from build123d import *

# Parameters (mm, degrees)
F0_R     = 2
F1_DEPTH = 4
F2_W     = 12
F2_H     = 4
F3_DEPTH = 4
F4_W     = 12
F4_H     = 20
F4_R     = 2
F5_DEPTH = 4


with BuildPart() as f1:
    # F0 (on Front) → F1 (new body)
    with BuildSketch(Plane.XZ):
        Polygon((-28, -4), (28, -4), (28, 4), (28, 16), (16, 16), (16, 4), (-16, 4), (-16, 16), (-28, 16), (-28, 4), align=None)
        with Locations((-24, 0)):
            Circle(F0_R, mode=Mode.SUBTRACT)
        Circle(F0_R, mode=Mode.SUBTRACT)
        with Locations((24, 0)):
            Circle(F0_R, mode=Mode.SUBTRACT)
    extrude(amount=-F1_DEPTH)

    # F2 (on face) → F3 (join)
    with BuildSketch(Plane.XZ):
        with Locations((22, 14)):
            Rectangle(F2_W, F2_H)
        with Locations((-22, 14)):
            Rectangle(F2_W, F2_H)
    extrude(amount=F3_DEPTH)

    # F4 (on face) → F5 (join)
    with BuildSketch(Plane.XZ.offset(4)):
        with Locations((22, 6)):
            Rectangle(F4_W, F4_H)
        with Locations((24, 0)):
            Circle(F4_R, mode=Mode.SUBTRACT)
        with Locations((-22, 6)):
            Rectangle(F4_W, F4_H)
        with Locations((-24, 0)):
            Circle(F4_R, mode=Mode.SUBTRACT)
    extrude(amount=F5_DEPTH)


solid = f1.part
Geometry: final body of the model. Coordinates: model frame, mm. A direction names the side the tool comes from. Coordinates: 2 decimals unless noted, no trailing zeros. Order: outer loops, then holes, each group sorted by start corner. A loop starts at its lowest first (then second) coordinate and runs counter-clockwise, first axis right, second up.
1) First-contact query: P1, Ø3, axis at x = -6, y = 1, coming from the +Z side; P2, Ø3, axis at x = -14, z = -0.5, coming from the -Y side; P3, Ø3, axis at x = 22, y = -2, coming from the -Z side. Flat tips, straight axial feed; report the tip coordinate or a pass-through.
Result sheet:
P1: stops at z = 4
P2: stops at y = 0
P3: stops at z = 12
2) Section C-C (z = 2.5). Return loops of the section in (x, y), then the cut area to 3 significant figures.
Result sheet:
outline: (-28, -8) - (-16, -8) - (-16, -4) - (-28, -4) - close; (-28, 0) - (28, 0) - (28, 4) - (-28, 4) - close; (16, -8) - (28, -8) - (28, -4) - (16, -4) - close
area: 320 mm2
3) Ray query, probe 1 along X at (y, z) = (-4.5, 12.5); probe 2 along Y at (x, z) = (-24, 3); probe 3 along Z at (x, y) = (24, 2.7). Return the intervals inside material, ascending.
Result sheet:
probe 1: x = -28 to -16, 16 to 28
probe 2: y = -8 to -4, 0 to 4
probe 3: z = -4 to -2, 2 to 16
4) Draft query along Y for faces 1 (the flat face through (-28, 1, 6)), 2 (the flat face through (-22, -4, 4)), 3 (the flat face through (-22, -8, 6)), 4 (the flat face through (22, -2, 12)). Return one class per face: released by +Y, released by -Y, zero draft, split by the parting line, or undercut.
Result sheet:
face 1: zero draft
face 2: undercut
face 3: released by -Y
face 4: undercut
5) Section D-D (y = 2.25). Return loops of the section in (x, z), then the cut area to 3 significant figures.
Result sheet:
outline: (-28, -4) - (28, -4) - (28, 16) - (16, 16) - (16, 4) - (-16, 4) - (-16, 16) - (-28, 16) - close; hole circle Ø4 at (-24, 0); hole circle Ø4 at (0, 0); hole circle Ø4 at (24, 0)
area: 698 mm2
6) Section B-B (x = -24). Return loops of the section in (y, z).
Result sheet:
outline: (-8, -4) - (-4, -4) - (-4, -2) - (-8, -2) - close; (-8, 2) - (-4, 2) - (-4, 12) - (0, 12) - (0, 2) - (4, 2) - (4, 16) - (-8, 16) - close; (0, -4) - (4, -4) - (4, -2) - (0, -2) - close
7) Set-up query: faces 5 (the flat face through (-7, 4, 2)), 6 (the flat face through (22, -4, 4)), 7 (the flat face through (-16, -5, 8)). Return all of +Z, -Z, +X, -X, +Y, -Y with unobstructed straight access to the full face (end or side cutting, diameter ignored); none if empty.
Result sheet:
face 5: +Z, -Z, +X, -X, +Y
face 6: -Z, +X, -X
face 7: +Z, -Y
8) Section A-A (y = -6.75). Return loops of the section in (x, z).
Result sheet:
outline: (-28, -4) - (-16, -4) - (-16, 16) - (-28, 16) - close; (16, -4) - (28, -4) - (28, 16) - (16, 16) - close; hole circle Ø4 at (-24, 0); hole circle Ø4 at (24, 0)
